Geometry: final body of the model. Coordinates: model frame, mm. A direction names the side the tool comes from. Round coordinates to 2 decimals unless told otherwise and drop trailing zeros. Loops run counter-clockwise (first coordinate to the right, second up) from the corner with the lowest first, then second, coordinate; pieces in that order, holes last. Notation, with made-up numbers: (51, 0.5) -> (94, 0.5) arc R20 ccw to (94, 21.5) -> close; hole circle Ø8 at (-14, 4.5). An arc over 180 degrees is marked (long way). Answer in a Markdown table with one row per item.
```python
from build123d import *

# Parameters (mm, degrees)
SKETCH1_W           = 25
SKETCH1_H           = 5
BOSS_EXTRUDE1_DEPTH = 2
SKETCH2_R           = 1.6
BOSS_EXTRUDE2_DEPTH = 4
SKETCH3_R           = 2.275
SKETCH3_R_2         = 1.6
BOSS_EXTRUDE3_DEPTH = 7.76


with BuildPart() as part:
    # Sketch1 → Boss-Extrude1 (new body)
    with BuildSketch(Plane.XY):
        with Locations((12.5, 2.5)):
            Rectangle(SKETCH1_W, SKETCH1_H)
    extrude(amount=BOSS_EXTRUDE1_DEPTH)

    # Sketch2 → Boss-Extrude2 (add)
    with BuildSketch(Plane.XY.offset(2)):
        with Locations((2.35, 2.5)):
            Circle(SKETCH2_R)
        with Locations((22.65, 2.5)):
            Circle(SKETCH2_R)
    extrude(amount=BOSS_EXTRUDE2_DEPTH)

    # Sketch3 → Boss-Extrude3 (add)
    # profile 1 of 2: a face of its own
    with BuildSketch(Plane(origin=(0, 0, 0), x_dir=(-1, 0, 0), z_dir=(0, 0, -1))):
        with Locations(Location((-20.47, 2.322974485, 0), (0, 0, 180))):
            Circle(SKETCH3_R)
        with Locations((-20.47, 2.322974485)):
            Circle(SKETCH3_R_2, mode=Mode.SUBTRACT)
    # profile 2 of 2: a face of its own
    with BuildSketch(Plane(origin=(0, 0, 0), x_dir=(-1, 0, 0), z_dir=(0, 0, -1))):
        with Locations(Location((-4.53, 2.322974485, 0), (0, 0, 180))):
            Circle(SKETCH3_R)
        with Locations((-4.53, 2.322974485)):
            Circle(SKETCH3_R_2, mode=Mode.SUBTRACT)
    extrude(amount=BOSS_EXTRUDE3_DEPTH)


solid = part.part
```
Item 1: Section query A-A, the plane z = 4.5. Output: boundary loops of the cut face in (x, y), and give its area (3 significant figures).
Ans:
| item | result |
|---|---|
| outline | circle Ø3.2 at (2.35, 2.5); circle Ø3.2 at (22.65, 2.5) |
| area | 16.1 mm2 |
Item 2: Section query B-B, the plane x = 20.47. Output: boundary loops of the cut face in (y, z), and give its area (3 significant figures).
Ans:
| item | result |
|---|---|
| outline | (0, 0) -> (0.05, 0) -> (0.05, -7.76) -> (0.72, -7.76) -> (0.72, 0) -> (3.92, 0) -> (3.92, -7.76) -> (4.6, -7.76) -> (4.6, 0) -> (5, 0) -> (5, 2) -> (0, 2) -> close |
| area | 20.5 mm2 |
Item 3: First-contact query: P1, Ø1.5, axis at x = 10.5, y = 3, coming from the +Z side; P2, Ø1, axis at y = 1.5, z = -5.5, coming from the -X side; P3, Ø1, axis at x = 21, y = 2.5, coming from the -Z side. Flat tips, straight axial feed; report the tip coordinate or a pass-through.
Ans:
| item | result |
|---|---|
| P1 | z = 2 |
| P2 | x = 2.28 |
| P3 | z = 0 |
Item 4: Section query C-C, the plane z = -3. Output: boundary loops of the cut face in (x, y) (3 decimals).
Ans:
| item | result |
|---|---|
| outline | circle Ø4.55 at (4.53, 2.323); circle Ø4.55 at (20.47, 2.323); hole circle Ø3.2 at (4.53, 2.323); hole circle Ø3.2 at (20.47, 2.323) |
Item 5: Set-up query: faces 5 (the cylindrical face through (3.83, 1.89, 3.97)), 6 (the flat face through (2, 3, 6)), 7 (the cylindrical face through (21.52, 4.34, -3.83)). Return all of +Z, -Z, +X, -X, +Y, -Y with unobstructed straight access to the full face (end or side cutting, diameter ignored); none if empty.
Ans:
| item | result |
|---|---|
| face 5 | +Z |
| face 6 | +Z, +X, -X, +Y, -Y |
| face 7 | -Z |
Item 6: Mould query, pull axis X, two halves, no side actions, for faces 1 (the flat face through (5, 2, 0)), 2 (the flat face through (21, 4, -7.76)), 3 (the cylindrical face through (24.176, 2.981, 3.972)), 4 (the flat face through (0, 2, 1)). Classes: released by +X, released by -X, zero draft, split by the parting line, or undercut.
Ans:
| item | result |
|---|---|
| face 1 | undercut |
| face 2 | zero draft |
| face 3 | undercut |
| face 4 | released by -X |
Item 7: Ray query, L1, parallel to Y at x = 4.53, z = -3; L2, parallel to X at y = 3.2, z = -0.5; L3, parallel to X at y = 2.4, z = 4.5. Return the intervals inside material, ascending.
Ans:
| item | result |
|---|---|
| L1 | 0.05 to 0.72, 3.92 to 4.6 |
| L2 | 2.43 to 3.19, 5.87 to 6.63, 18.37 to 19.13, 21.81 to 22.57 |
| L3 | 0.75 to 3.95, 21.05 to 24.25 |
Item 8: Section query D-D, the plane y = 3.65. Output: boundary loops of the cut face in (x, z).
Ans:
| item | result |
|---|---|
| outline | (0, 0) -> (2.68, 0) -> (2.68, -7.76) -> (3.64, -7.76) -> (3.64, 0) -> (5.42, 0) -> (5.42, -7.76) -> (6.38, -7.76) -> (6.38, 0) -> (18.62, 0) -> (18.62, -7.76) -> (19.58, -7.76) -> (19.58, 0) -> (21.36, 0) -> (21.36, -7.76) -> (22.32, -7.76) -> (22.32, 0) -> (25, 0) -> (25, 2) -> (23.76, 2) -> (23.76, 6) -> (21.54, 6) -> (21.54, 2) -> (3.46, 2) -> (3.46, 6) -> (1.24, 6) -> (1.24, 2) -> (0, 2) -> close |
